Design review of the part shown in the three views and the two pictorial views. Dimensions are in mm from the part's minimum x, y and z. Give positions to 0.01 mm unless a question says otherwise; leave off trailing zeros. Loops run counter-clockwise (first coordinate to the right, second up) from the corner with the lowest first, then second, coordinate; pieces in that order, holes last.
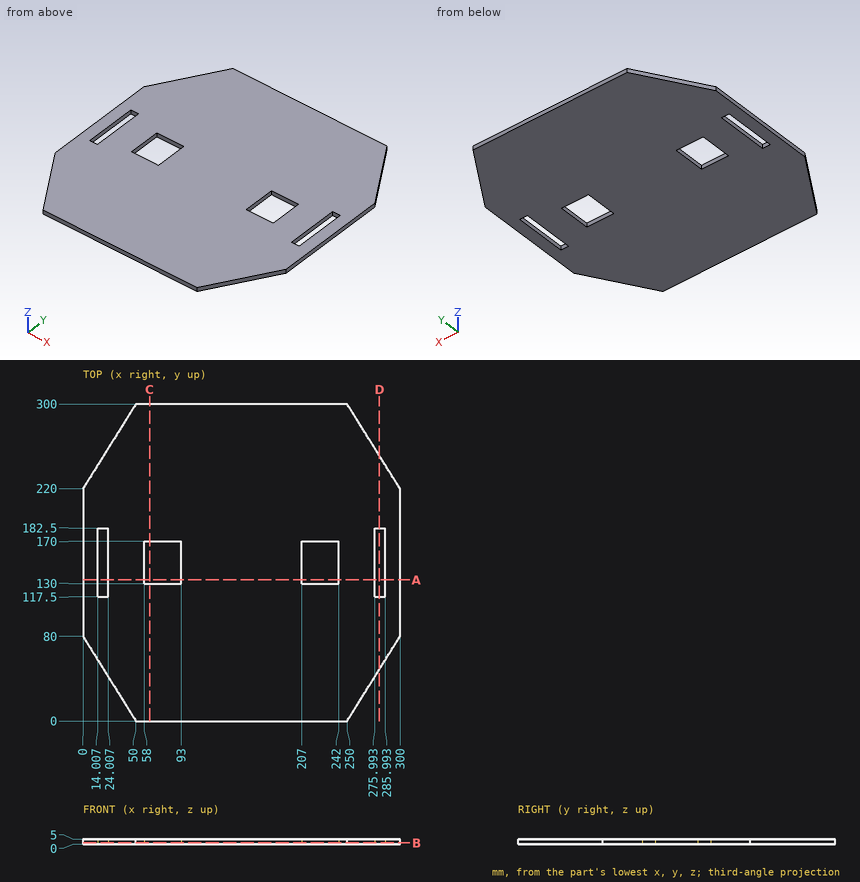
Q1. Consider section C-C on x = 63. Give the boundary of the cut face in (y, z).
Answers:
outline: (0, 0) - (130, 0) - (130, 5) - (0, 5) - close; (170, 0) - (300, 0) - (300, 5) - (170, 5) - close
Q2. Consider section A-A on y = 133.5. Give the boundary of the cut face in (x, z).
Answers:
outline: (0, 0) - (14.01, 0) - (14.01, 5) - (0, 5) - close; (24.01, 0) - (58, 0) - (58, 5) - (24.01, 5) - close; (93, 0) - (207, 0) - (207, 5) - (93, 5) - close; (242, 0) - (275.99, 0) - (275.99, 5) - (242, 5) - close; (285.99, 0) - (300, 0) - (300, 5) - (285.99, 5) - close
Q3. For probe 1 along X at (y, z) = (166.5, 2.2); probe 2 along X at (y, z) = (118, 2); probe 3 along Y at (x, z) = (227.5, 1.9), list the stretches that pass through material, from the lowest coordinate up.
Answers:
probe 1: x = 0 to 14.01, 24.01 to 58, 93 to 207, 242 to 275.99, 285.99 to 300
probe 2: x = 0 to 14.01, 24.01 to 275.99, 285.99 to 300
probe 3: y = 0 to 130, 170 to 300
Q4. Consider section B-B on z = 1.4. Give the boundary of the cut face in (x, y).
Answers:
outline: (0, 80) - (50, 0) - (250, 0) - (300, 80) - (300, 220) - (250, 300) - (50, 300) - (0, 220) - close; hole (14.01, 117.5) - (24.01, 117.5) - (24.01, 182.5) - (14.01, 182.5) - close; hole (58, 130) - (93, 130) - (93, 170) - (58, 170) - close; hole (207, 130) - (242, 130) - (242, 170) - (207, 170) - close; hole (275.99, 117.5) - (285.99, 117.5) - (285.99, 182.5) - (275.99, 182.5) - close
Q5. For pin 1 Ø1.5 at (x, z) = (280.5, 3) entering from -Y; pin 2 Ø1 at (y, z) = (263.5, 3.5) entering from +X (1 decimal), all flat-tipped, find the tip position at first contact; note any pin that passes through.
Answers:
pin 1: stops at y = 47.6
pin 2: stops at x = 273.1
Q6. Consider section D-D on x = 280.5. Give the boundary of the cut face in (y, z).
Answers:
outline: (48.8, 0) - (117.5, 0) - (117.5, 5) - (48.8, 5) - close; (182.5, 0) - (251.2, 0) - (251.2, 5) - (182.5, 5) - close
